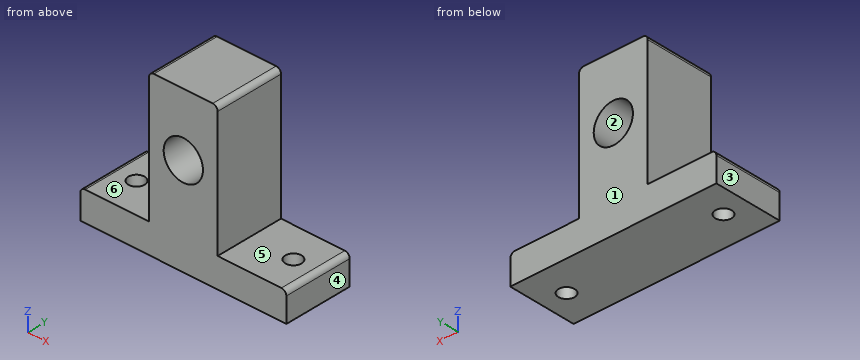
from build123d import *

# Parameters (mm, degrees)
F0_R     = 4
F1_DEPTH = 14
F3_D     = 3.3


with BuildPart() as f1:
    # F0 (on Front) → F1 (new body)
    with BuildSketch(Plane.XZ):
        with BuildLine():
            Line((20, -14), (7, -14))
            Line((7, -14), (7, 11.8))
            ThreePointArc((7, 11.8), (6.707107, 12.507107), (6, 12.8))
            Line((6, 12.8), (-6, 12.8))
            ThreePointArc((-6, 12.8), (-6.707107, 12.507107), (-7, 11.8))
            Line((-7, 11.8), (-7, -14))
            Line((-7, -14), (-20, -14))
            ThreePointArc((-20, -14), (-20.707107, -14.292893), (-21, -15))
            Line((-21, -15), (-21, -20))
            Line((-21, -20), (21, -20))
            Line((21, -20), (21, -15))
            ThreePointArc((21, -15), (20.707107, -14.292893), (20, -14))
        make_face()
        Circle(F0_R, mode=Mode.SUBTRACT)
    extrude(amount=F1_DEPTH)

    # F3 (through all)
    with Locations(Plane.XY):
        with Locations((-16, -7), (16, -7)):
            Hole(F3_D / 2)


solid = f1.part
Design review of the part built by this model. Coordinates are the model's own, in mm. Face numbers are marked on the shaded views. A direction names the side the tool comes from. Coordinates: 2 decimals unless noted, no trailing zeros. Order: outer loops, then holes, each group sorted by start corner. A loop starts at its lowest first (then second) coordinate and runs counter-clockwise, first axis right, second up. Notation, with made-up numbers: (68.5, 67.5) -> (85.5, 67.5) arc R17 cw to (85.5, 83.5) -> close; hole circle Ø4 at (49, -14). An arc over 180 degrees is marked (long way). Use one line per item in the form item = value. Start each with the question number.
(1) Add section C-C on z = 0. State the section outline as (x, y) points, plus the area to 3 significant figures.
(2) For probe 1 along Y at (x, z) = (16, -18); probe 2 along X at (y, z) = (-9.25, 0.5); probe 3 along Z at (x, y) = (0, -10.25), list the stretches that pass through material, from the lowest coordinate up.
(3) The part is to be moulded in two halves that separate along X. For the marked faces 1, 2 and 3, say which applies: +X half, -X half, draft (parallel to the pull), parting line (faces both ways), or undercut.
(4) Add section D-D on y = -9.5. State the section outline as (x, z) points, plus the area to 3 significant figures.
(5) For the marked faces 4, 5 and 6, list the 3-axis set-ups (+Z, -Z, +X, -X, +Y, -Y) from which the entire face can be reached by the end or side of a thin tool; tool diameter is ignored.
(6) Insertion check: pin 1 (4 mm diameter, centred on y = -6, z = -1.5, fed in from -X); pin 2 (4 mm diameter, centred on x = 0, z = 3.5, fed in from -Y); pin 3 (6.5 mm diameter, centred on x = 13, y = -6.5, fed in from +Z); pin 4 (5 mm diameter, centred on y = -5.5, z = 1, fed in from +X). Each pin has a flat end and moves straight along its axis. Give the tip position at first contact, or say it passes through.
(7) Add section B-B on x = 0. State the section outline as (y, z) points, plus the area to 3 significant figures.
(8) Add section A-A on y = -7. State the section outline as (x, z) points, plus the area to 3 significant figures.
Answer block:
q1.outline = (-7, -14) -> (-4, -14) -> (-4, 0) -> (-7, 0) -> close; (4, -14) -> (7, -14) -> (7, 0) -> (4, 0) -> close
q1.area = 84.0 mm²
q2.probe_1 = -14 to -8.65, -5.35 to 0
q2.probe_2 = -7 to -3.97, 3.97 to 7
q2.probe_3 = -20 to -4, 4 to 12.8
q3.face_1 = draft
q3.face_2 = undercut
q3.face_3 = -X half
q4.outline = (-21, -20) -> (21, -20) -> (21, -15) arc R1 ccw to (20, -14) -> (7, -14) -> (7, 11.8) arc R1 ccw to (6, 12.8) -> (-6, 12.8) arc R1 ccw to (-7, 11.8) -> (-7, -14) -> (-20, -14) arc R1 ccw to (-21, -15) -> close; hole circle Ø8 at (0, 0)
q4.area = 576 mm²
q5.face_4 = +Z, -Z, +X, +Y, -Y
q5.face_5 = +Z, +X, +Y, -Y
q5.face_6 = +Z, -X, +Y, -Y
q6.pin_1 = -7
q6.pin_2 = -14
q6.pin_3 = -14
q6.pin_4 = 7
q7.outline = (-14, -20) -> (0, -20) -> (0, -4) -> (-14, -4) -> close; (-14, 4) -> (0, 4) -> (0, 12.8) -> (-14, 12.8) -> close
q7.area = 347 mm²
q8.outline = (-21, -20) -> (-17.65, -20) -> (-17.65, -14) -> (-20, -14) arc R1 ccw to (-21, -15) -> close; (-14.35, -20) -> (14.35, -20) -> (14.35, -14) -> (7, -14) -> (7, 11.8) arc R1 ccw to (6, 12.8) -> (-6, 12.8) arc R1 ccw to (-7, 11.8) -> (-7, -14) -> (-14.35, -14) -> close; (17.65, -20) -> (21, -20) -> (21, -15) arc R1 ccw to (20, -14) -> (17.65, -14) -> close; hole circle Ø8 at (0, 0)
q8.area = 536 mm²
